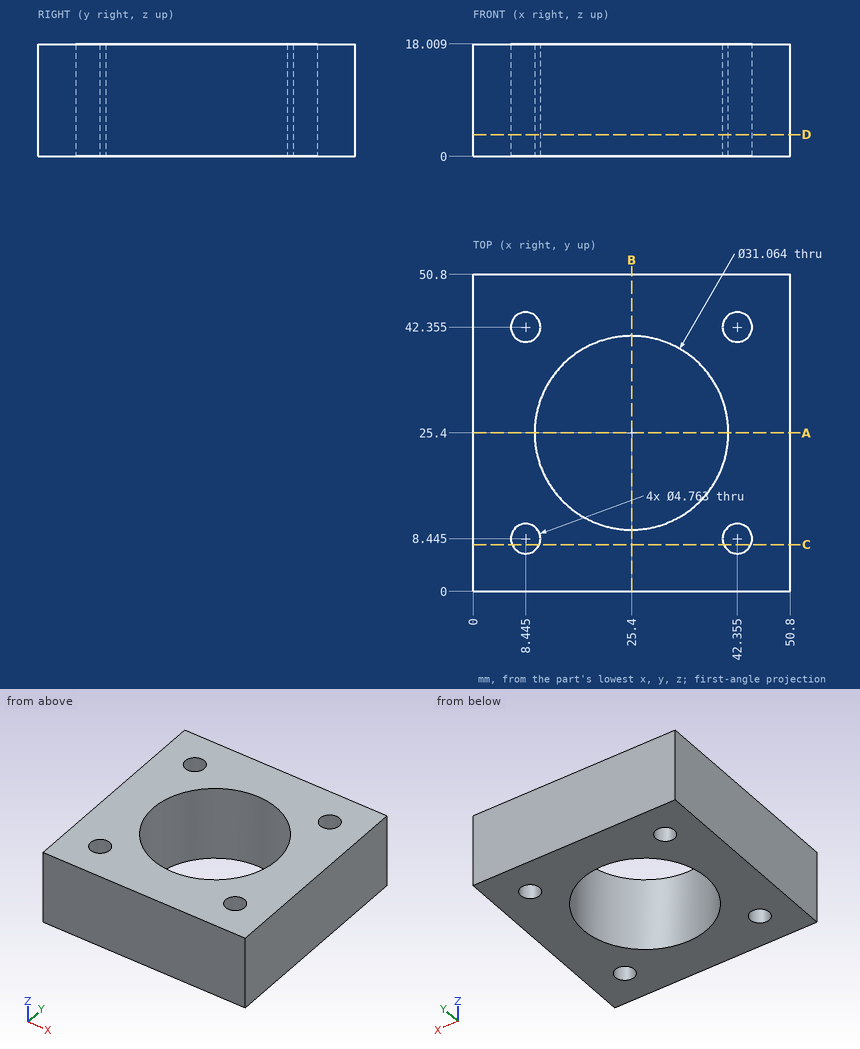
Could you check a few things on this drawing? It's one solid part, dimensions in mm from its lowest x, y, z. Coordinates: 2 decimals unless noted, no trailing zeros. Loops run counter-clockwise (first coordinate to the right, second up) from the corner with the lowest first, then second, coordinate; pieces in that order, holes last.
1. Imagine slicing it at A-A (y = 25.4). Please give me the cut outline in (x, z).
2. Imagine slicing it at D-D (z = 3.5). Please give me the cut outline in (x, y) (1 decimal), and give its area (3 significant figures).
3. Imagine slicing it at C-C (y = 7.5). Please give me the cut outline in (x, z).
4. I need wall thicknesses on L1, parallel to X at y = 8.5, z = 12.25 (1 decimal); L2, parallel to Y at x = 25.4, z = 4; L3, parallel to X at y = 20, z = 5. Which ranges of each line are inside material? Lowest first, please.
5. For P1, Ø3, axis at x = 42.35, y = 8.45, coming from the +Z side, with a flat end and sliding along its axis, tell me the tip position at first contact or that it passes through.
Computed values:
1. outline: (0, 0) - (9.87, 0) - (9.87, 18.01) - (0, 18.01) - close; (40.93, 0) - (50.8, 0) - (50.8, 18.01) - (40.93, 18.01) - close
2. outline: (0, 0) - (50.8, 0) - (50.8, 50.8) - (0, 50.8) - close; hole circle Ø4.8 at (8.4, 8.4); hole circle Ø4.8 at (8.4, 42.4); hole circle Ø31.1 at (25.4, 25.4); hole circle Ø4.8 at (42.4, 8.4); hole circle Ø4.8 at (42.4, 42.4)
2. area: 1,750 mm2
3. outline: (0, 0) - (6.26, 0) - (6.26, 18.01) - (0, 18.01) - close; (10.63, 0) - (40.17, 0) - (40.17, 18.01) - (10.63, 18.01) - close; (44.54, 0) - (50.8, 0) - (50.8, 18.01) - (44.54, 18.01) - close
4. L1: x = 0 to 6.1, 10.8 to 40, 44.7 to 50.8
4. L2: y = 0 to 9.87, 40.93 to 50.8
4. L3: x = 0 to 10.84, 39.96 to 50.8
5. P1: passes through
